Verification items for the finished model (mm, model axes). A direction names the side the tool comes from. Give positions to 0.01 mm unless a question says otherwise; leave off trailing zeros. Write each loop counter-clockwise with the first axis right and the second up, starting at its lowest first coordinate (ties: lowest second). Pieces come first, ordered by that corner, then holes. Notation, with made-up numbers: (53.5, 20.5) -> (86.5, 20.5) arc R22 ccw to (86.5, 54.5) -> close; hole circle Ø9 at (44, -27.75). An arc over 180 degrees is marked (long way). Answer as CSV lines item,"result". Start each with the question number.
1) Material ranges on L1, parallel to Y at x = -2.15, z = -11; L2, parallel to X at y = 35, z = -11, recorded low to high.
2) Mould release check, pull along X, two halves, no side actions. Record for faces 3 (the cylindrical face through (-21, 32, -20)), 4 (the cylindrical face through (-15.76, 32.96, -7.35)), 5 (the flat face through (-11, 30, 0)): released by +X, released by -X, zero draft, split by the parting line, or undercut.
3) Tool access check on faces 1 (the flat face through (-22, 32, -9)), 2 (the cylindrical face through (-2.68, 7.23, -10.71)). Record the directions out of +Z, -Z, +X, -X, +Y, -Y that give a thin tool (end or side, any length) a straight path to the whole face; none if there is none.
4) Sectioned sample at C-C on x = -10.25. Record the cut outline in (y, z), and give its area (3 significant figures).
5) Sectioned sample at B-B on z = -11. Record the cut outline in (x, y).
6) Sectioned sample at D-D on y = 5. Record the cut outline in (x, z), and give its area (3 significant figures).
7) Sectioned sample at A-A on y = 37. Record the cut outline in (x, z), and give its area (3 significant figures).
8) Gauge pin test, flat ends, axial feed: pin 1 Ø1 at (y, z) = (38, -18) entering from +X; pin 2 Ø4 at (x, z) = (-6, -17.5) entering from -Y; pin 3 Ø3.5 at (y, z) = (60, -11) entering from +X. Record the tip position at first contact, or that the pin passes through.
Autodesk Inventor part; units mm, degrees
ref_plane "YZ-Ebene" through (0, 0, 0) normal (1, 0, 0) x (0, 1, 0)
ref_plane "XZ-Ebene" through (0, 0, 0) normal (0, 1, 0) x (-1, 0, 0)
ref_plane "XY-Ebene" through (0, 0, 0) normal (0, 0, 1) x (1, 0, 0)
sketch "Skizze1" plane through (0, 0, 0) normal (0, 1, 0) x (-1, 0, 0)
  line L0 (22, 0) -> (0, 0)
  line L1 (0, 0) -> (0, -17)
  line L2 (5, -22) -> (17, -22)
  line L3 (22, -17) -> (22, 0)
  arc A0 (17, -22) -> (22, -17) centre (17, -17) ccw
  arc A1 (0, -17) -> (5, -22) centre (5, -17) ccw
  point P0 (0, 0)
  point P1 (22, 0)
  point P2 (0, -22)
  point P3 (0, 0)
  point P4 (22, -22)
  point P5 (0, 0)
  point P6 (0, 0)
  point P7 (0, 0)
  point P8 (22, 0)
  point P9 (22, 0)
  point P10 (22, 0)
  point P11 (0, -22)
  point P12 (0, -22)
  point P13 (0, -22)
  point P14 (22, 0)
  dimension "d0" = 22
  dimension "d1" = 22
  dimension "d32" = 5
  dimension "d37" = 5
extrude "Extrusion1" add sketch "Skizze1" along normal blind 65
sketch "Skizze2" plane through (0, 65, 0) normal (0, 1, 0) x (1, 0, 0)
  circle A0 centre (-11, 11) radius 6
  line L0 (-5, 22) -> (-17, 22)
  line L1 (0, 0) -> (0, 17)
  point P0 (0, 22)
  point P1 (-22, 22)
  point P2 (0, 22)
  dimension "d6" = 12
  dimension "d17" = 11
  dimension "d18" = 11
extrude "Extrusion2" cut sketch "Skizze2" against normal blind 84
sketch "Skizze3" plane through (0, 0, 0) normal (1, 0, 0) x (0, 0, -1)
  circle A0 centre (11, 60) radius 2.25
  circle A1 centre (11, 5) radius 2.25
  line L0 (22, 0) -> (22, 65)
  line L1 (0, 0) -> (17, 0)
  line L2 (0, 0) -> (0, 84)
  point P0 (22, 0)
  dimension "d11" = 5
  dimension "d12" = 55
  dimension "d13" = 4.5
  dimension "d14" = 4.5
  dimension "d28" = 11
  dimension "d29" = 11
extrude "Extrusion3" cut sketch "Skizze3" against normal blind 12
sketch "Skizze6" plane through (-22, 0, -17) normal (-1, 0, 0) x (0, 0, 1)
  line L0 (0, 0) -> (17, 0)
  line L1 (0, 65) -> (-5, 65)
  line L2 (12, 0) -> (-5, 0)
  line L3 (-5, 0) -> (-5, 65)
  line L4 (-5, 65) -> (12, 65)
  line L5 (17, 60) -> (17, 5)
  arc A0 (17, 60) -> (12, 65) centre (12, 60) ccw
  line L6 (17, 0) -> (-5, 0)
  line L7 (-5, 0) -> (-5, 65)
  line L8 (-5, 65) -> (17, 65)
  line L9 (17, 65) -> (17, 0)
  point P0 (12, 65)
  dimension "d33" = 5
extrude "Extrusion5" cut sketch "Skizze6" against normal blind 25 contours A0 L8 L9
properties part number "microscope_mount"
Ans:
1,L1,"y = 0 to 2.75, 7.25 to 57.75, 62.25 to 65"
1,L2,"x = -22 to -17, -5 to 0"
2,face 3,"released by -X"
2,face 4,"undercut"
2,face 5,"zero draft"
3,face 1,"+Z, -Z, -X, +Y, -Y"
3,face 2,"+X"
4,outline,"(0, -22) -> (65, -22) -> (65, -16.95) -> (0, -16.95) -> close; (0, -5.05) -> (65, -5.05) -> (65, -5) arc R5 ccw to (60, 0) -> (0, 0) -> close"
4,area,"651 mm²"
5,outline,"(-22, 0) -> (-17, 0) -> (-17, 65) -> (-22, 65) -> close; (-5, 0) -> (0, 0) -> (0, 2.75) -> (-5, 2.75) -> close; (-5, 7.25) -> (0, 7.25) -> (0, 57.75) -> (-5, 57.75) -> close; (-5, 62.25) -> (0, 62.25) -> (0, 65) -> (-5, 65) -> close"
6,outline,"(-22, -17) arc R5 ccw to (-17, -22) -> (-5, -22) arc R5 ccw to (0, -17) -> (0, -13.25) -> (-5.44, -13.25) arc R6 cw (long way) to (-5.44, -8.75) -> (0, -8.75) -> (0, 0) -> (-22, 0) -> close"
6,area,"337 mm²"
7,outline,"(-22, -17) arc R5 ccw to (-17, -22) -> (-5, -22) arc R5 ccw to (0, -17) -> (0, 0) -> (-22, 0) -> close; hole circle Ø12 at (-11, -11)"
7,area,"360 mm²"
8,pin 1,"stops at x = -0.03"
8,pin 2,"stops at y = 0"
8,pin 3,"stops at x = -16.74"
